For this review, take the finished solid that the model builds, in its own axes (mm). A direction names the side the tool comes from. Coordinates: 2 decimals unless noted, no trailing zeros. Write each loop counter-clockwise with the first axis right and the second up, starting at its lowest first coordinate (ties: lowest second). Pieces come first, ordered by that corner, then holes.
```python
from build123d import *

# Parameters (mm, degrees)
F0_R     = 26.035
F0_R_2   = 22.86
F1_DEPTH = 50.8
F0_R_3   = 3.556
F2_DEPTH = 6.35


with BuildPart() as f1:
    # F0 (on Top) → F1 (new body)
    with BuildSketch(Plane.XY):
        Circle(F0_R)
        Circle(F0_R_2, mode=Mode.SUBTRACT)
    extrude(amount=F1_DEPTH)

    # F0 (on Top) → F2 (join)
    with BuildSketch(Plane.XY):
        with BuildLine():
            Line((26.150901, 28.575), (-26.150901, 28.575))
            ThreePointArc((-26.150901, 28.575), (-38.735, 0), (-26.150901, -28.575))
            Line((-26.150901, -28.575), (26.150901, -28.575))
            ThreePointArc((26.150901, -28.575), (38.735, 0), (26.150901, 28.575))
        make_face()
        with Locations((-32.804761, 0)):
            Circle(F0_R_3, mode=Mode.SUBTRACT)
        Circle(F0_R, mode=Mode.SUBTRACT)
        with Locations((32.804761, 0)):
            Circle(F0_R_3, mode=Mode.SUBTRACT)
    extrude(amount=F2_DEPTH)


solid = f1.part
```
Q1. Add section B-B (x = 0). State the section outline as (y, z) points (3 decimals), then the cut area to 3 significant figures.
Ans:
outline: (-28.575, 0) - (-22.86, 0) - (-22.86, 50.8) - (-26.035, 50.8) - (-26.035, 6.35) - (-28.575, 6.35) - close; (22.86, 0) - (28.575, 0) - (28.575, 6.35) - (26.035, 6.35) - (26.035, 50.8) - (22.86, 50.8) - close
area: 355 mm2
Q2. For probe 1 along Y at (x, z) = (-1.5, 8); probe 2 along Z at (x, y) = (29, -25.5); probe 3 along X at (y, z) = (-9, 31), list the stretches that pass through material, from the lowest coordinate up.
Ans:
probe 1: y = -25.99 to -22.81, 22.81 to 25.99
probe 2: z = 0 to 6.35
probe 3: x = -24.43 to -21.01, 21.01 to 24.43
Q3. Draft analysis for pull direction X (two halves, no side actions). For faces 3 (the flat face through (-0.12, -23.02, 50.8)), 4 (the cylindrical face through (38.732, -0.45, 3.131)), 5 (the cylindrical face through (-38.732, 0.45, 3.131)), 6 (the cylindrical face through (-36.357, 0.156, 3.131)), state which applies: +X half, -X half, draft (parallel to the pull), parting line (faces both ways), or undercut.
Ans:
face 3: draft
face 4: +X half
face 5: -X half
face 6: undercut
Q4. Add section C-C (y = 0). State the section outline as (x, z) points (3 decimals), then the cut area to 3 significant figures.
Ans:
outline: (-38.735, 0) - (-36.361, 0) - (-36.361, 6.35) - (-38.735, 6.35) - close; (-29.249, 0) - (-22.86, 0) - (-22.86, 50.8) - (-26.035, 50.8) - (-26.035, 6.35) - (-29.249, 6.35) - close; (22.86, 0) - (29.249, 0) - (29.249, 6.35) - (26.035, 6.35) - (26.035, 50.8) - (22.86, 50.8) - close; (36.361, 0) - (38.735, 0) - (38.735, 6.35) - (36.361, 6.35) - close
area: 394 mm2
Q5. Tool access review of faces 1 (the flat face through (0, -28.575, 3)), 2 (the flat face through (-26.4, 0.4, 6.35)): name each direction out of +Z, -Z, +X, -X, +Y, -Y from which nothing blocks a thin tool from reaching the whole face with its end or side.
Ans:
face 1: +Z, -Z, +X, -X, -Y
face 2: +Z
Q6. Add section A-A (z = 4.5). State the section outline as (x, y) points (3 decimals).
Ans:
outline: (-26.151, -28.575) - (26.151, -28.575) arc R38.735 ccw to (26.151, 28.575) - (-26.151, 28.575) arc R38.735 ccw to start; hole circle Ø7.112 at (-32.805, 0); hole circle Ø45.72 at (0, 0); hole circle Ø7.112 at (32.805, 0)
Q7. Add section D-D (y = -13). State the section outline as (x, z) points, then the cut area to 3 significant figures.
Ans:
outline: (-36.49, 0) - (-18.8, 0) - (-18.8, 50.8) - (-22.56, 50.8) - (-22.56, 6.35) - (-36.49, 6.35) - close; (18.8, 0) - (36.49, 0) - (36.49, 6.35) - (22.56, 6.35) - (22.56, 50.8) - (18.8, 50.8) - close
area: 558 mm2
Q8. Clearance check with flat-ended pins moving along their axes: pin 1 Ø1 at (x, z) = (23.5, 17) entering from +Y; pin 2 Ø3 at (y, z) = (-20, 19) entering from -X; pin 3 Ø6 at (y, z) = (10, 26.5) entering from -X; pin 4 Ø10 at (x, y) = (22, 21) entering from -Z. State where each tip first meets the part, or that it passes through.
Ans:
pin 1: stops at y = 12.2
pin 2: stops at x = -18.32
pin 3: stops at x = -25.08
pin 4: stops at z = 0
